For this review, take the finished solid that the model builds, in its own axes (mm). A direction names the side the tool comes from. Coordinates: 2 decimals unless noted, no trailing zeros. Write each loop counter-clockwise with the first axis right and the second up, starting at its lowest first coordinate (ties: lowest second). Pieces come first, ordered by that corner, then holes. Notation, with made-up numbers: (67, 79.25) -> (98, 79.25) arc R18 cw to (98, 96.25) -> close; hole circle Ø5 at (57, -9). An arc over 180 degrees is marked (long way). Put each result on its own line as item: value. Start each with the question number.
Item 1: The part is to be moulded in two halves that separate along X. For faces 4 (the cylindrical face through (5.662, -0.748, -1.438)), 5 (the cylindrical face through (55.822, -2.373, -3.095)), 6 (the conical face through (0.14, -3.64, -0.05)), say which applies: +X half, -X half, draft (parallel to the pull), parting line (faces both ways), or undercut.
Item 2: Consider section B-B on x = 20.5. Give the boundary of the cut face in (y, z), and give its area (3 significant figures).
Item 3: Consider section A-A on x = 9.5. Give the boundary of the cut face in (y, z), and give its area (3 significant figures).
Item 4: For faces 1 (the flat face through (51.4, -3, -3)), 2 (the cylindrical face through (65.006, -2.373, -3.095)), 3 (the flat face through (57.4, -3, -3)), list the 3-axis set-ups (+Z, -Z, +X, -X, +Y, -Y) from which the entire face can be reached by the end or side of a thin tool; tool diameter is ignored.
Item 5: Insertion check: P1, Ø6, axis at x = 25.5, y = -5, coming from the -Z side; P2, Ø5, axis at x = 18.5, y = 3.5, coming from the +Z side; P3, Ø4, axis at x = 43, z = 1, coming from the -Y side. Each pin has a flat end and moves straight along its axis. Give the tip position at first contact, or say it passes through.
Item 6: To check wall thickness, follow L1, parallel to X at y = -6, z = 3.25; L2, parallel to Z at x = 6.5, y = 0; L3, parallel to X at y = 3, z = 3.75. State the ranges of each line that lie inside material, in increasing order.
```python
from build123d import *

# Parameters (mm, degrees)
CUT_EXTRUDE_1_DEPTH      = 8
CUT_EXTRUDE_1_DEPTH_BACK = 8


with BuildPart() as part:
    # Sketch 1 → Revolve 1 (revolve)
    with BuildSketch(Plane.XY, mode=Mode.PRIVATE) as revolve_1_sk:
        Polygon((0, 0), (0, 3.5), (0.5, 4), (51.4, 4), (51.4, 7.6), (51.6, 7.8), (54, 7.8), (54.2, 7.6), (54.2, 3.9), (57.4, 3.9), (57.4, 7.6), (57.6, 7.8), (58.4, 7.8), (58.6, 7.6), (58.6, 5.7), (60.4, 5.7), (60.4, 7.6), (60.6, 7.8), (61.1, 7.8), (61.3, 7.6), (61.3, 7.2), (63.6, 7.2), (63.6, 7.6), (63.8, 7.8), (64.4, 7.8), (64.6, 7.6), (64.6, 3.9), (65.4, 3.9), (65.6, 3.7), (65.6, 0), align=None)
    revolve(revolve_1_sk.sketch.rotate(Axis((65.6, 0, 0), (-1, 0, 0)), 270), axis=Axis((65.6, 0, 0), (-1, 0, 0)))

    # Sketch 2 → Cut-Revolve 1 (revolve, cut)
    with BuildSketch(Plane.XY, mode=Mode.PRIVATE) as cut_revolve_1_sk:
        Polygon((0, 0), (0, 2), (0.379, 1.621), (10.8, 1.621), (11.735884786, 0), align=None)
    revolve(cut_revolve_1_sk.sketch.rotate(Axis((11.735884786, 0, 0), (-1, 0, 0)), 180), axis=Axis((11.735884786, 0, 0), (-1, 0, 0)), mode=Mode.SUBTRACT)

    # Sketch 3 → Cut-Extrude 1 (cut, two sides: drawn at the far end of the back side and taken through both)
    with BuildSketch(Plane(origin=(0, 0, 0), x_dir=(1, 0, 0), z_dir=(0, 1, 0)).offset(-CUT_EXTRUDE_1_DEPTH_BACK)):
        Polygon((-9.2, -10.121067812), (10.071067812, -10.121067812), (3, -3.05), (0, -3.05), (0, 3.05), (3, 3.05), (10.071067812, 10.121067812), (-9.2, 10.121067812), align=None)
    extrude(amount=CUT_EXTRUDE_1_DEPTH + CUT_EXTRUDE_1_DEPTH_BACK, mode=Mode.SUBTRACT)


solid = part.part
```
Return value:
1. face 4: draft
1. face 5: undercut
1. face 6: -X half
2. outline: circle Ø8 at (0, 0)
2. area: 50.3 mm^2
3. outline: circle Ø8 at (0, 0); hole circle Ø3.24 at (0, 0)
3. area: 42.0 mm^2
4. face 1: -X
4. face 2: +X
4. face 3: none
5. P1: z = -3.46
5. P2: z = 3.87
5. P3: y = -4
6. L1: 51.4 to 54.2, 57.4 to 58.6, 60.4 to 64.6
6. L2: -4 to -1.62, 1.62 to 4
6. L3: 51.4 to 54.2, 57.4 to 64.6
